Here's how the part is built. I have some questions about the finished solid (model axes, mm). Face numbers are marked on the shaded views. A direction names the side the tool comes from. Coordinates: 2 decimals unless noted, no trailing zeros. Loops run counter-clockwise (first coordinate to the right, second up) from the corner with the lowest first, then second, coordinate; pieces in that order, holes last. Notation, with made-up numbers: M 35,23.25 L 63,23.25 A25 ccw 63,62.25 Z; hole C 7,-13.5 d11. An arc over 180 degrees is marked long. Use CSV: the item, a comma, the result in double quotes. Start each with the question number.
Q1. If we section it at D-D (z = 2.75): Please give me the cut outline in (x, y).
Q2. Which directions (+Z, -Z, +X, -X, +Y, -Y) give clear straight access to the entire face, cutting with the end or side of a thin tool? Please do the marked faces 1 and 2.
Q3. If we section it at C-C (y = 6.25): Please give me the cut outline in (x, z) (3 decimals), and give its area (3 significant figures).
Q4. If we section it at A-A (y = 3.5): Please give me the cut outline in (x, z) (3 decimals), and give its area (3 significant figures).
Q5. If we mould it in two halves opening along Y, with no side actions, what happens to the marked faces 3, 4 and 5? For each: +Y half, -Y half, draft (parallel to the pull), parting line (faces both ways), or undercut.
Q6. For pin 1 Ø3.5 at (y, z) = (5, 16.5) entering from -X; pin 2 Ø5 at (x, y) = (6.5, 4) entering from +Z; pin 3 Ø2.5 at (x, z) = (36.5, 3.5) entering from +Y, each with a flat end and sliding along its axis, tell me the tip position at first contact or that it passes through.
Q7. Please list where these lines run through material, in increasing order: probe 1 along Z at (x, y) = (36.5, 5.5) (3 decimals); probe 2 along Z at (x, y) = (36.5, 6.5) (3 decimals); probe 3 along X at (y, z) = (3.5, 5.75). Write a range as [from, to].
Q8. If we section it at B-B (x = 36.5): Please give me the cut outline in (y, z) (3 decimals), and give its area (3 significant figures).
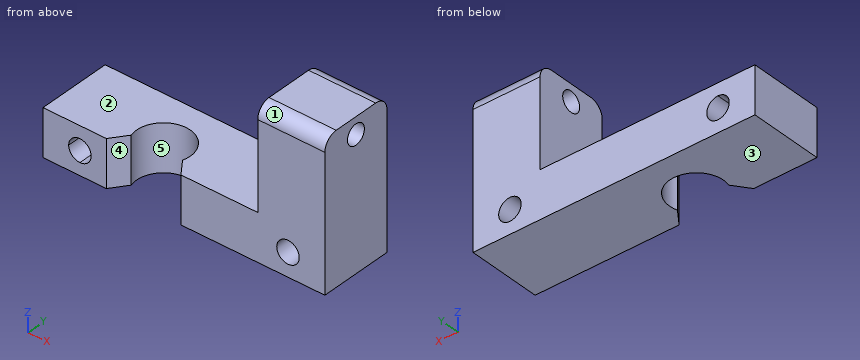
from build123d import *

# Parameters (mm, degrees)
F1_W        = 42
F1_H        = 11
F2_DEPTH    = 7
F3_R        = 4
F4_DEPTH    = 25
F5_T1_DEPTH = 25.9605224852
F7_DEPTH    = 25
F8_W        = 10
F8_H        = 11
F9_DEPTH    = 15
F10_R       = 1.5
F11_DEPTH   = 25
F12_R       = 2


# Not quite as in the source:
# - a fillet or chamfer that OpenCascade refuses, or shapes differently, is made with other operations: its cross-section is extruded or revolved along the edge and cut away or added


with BuildPart() as f2:
    # F1 (on Top) → F2 (new body)
    with BuildSketch(Plane.XY):
        with Locations((21, 5.5)):
            Rectangle(F1_W, F1_H)
    extrude(amount=F2_DEPTH)

    # F3 (on face) → F4 (cut)
    with BuildSketch(Plane.XY.offset(7)):
        with Locations((15, 3.5)):
            Circle(F3_R)
    extrude(amount=-F4_DEPTH, mode=Mode.SUBTRACT)

    # F5: chamfer of 7 on 2 edges, made by hand

    # F5_s2 → F5_t1 (cut)
    with BuildSketch(Plane.XY.offset(-9.4802612426)):
        with BuildLine():
            Line((20.721915214, -0.225000294), (18.6596772309, 2.5591704653))
            Line((18.6596772309, 2.5591704653), (18.5257555, 2.5999745093))
            ThreePointArc((18.5257555, 2.5999745093), (18.0236462707, 1.1005910665), (16.8687144645, 0.1225))
            Line((16.8687144645, 0.1225), (16.9364916731, -0.14))
            ThreePointArc((16.9364916731, -0.14), (18.8292034436, -0.14), (20.721915214, -0.365000294))
            Line((20.721915214, -0.365000294), (20.721915214, -0.225000294))
        make_face()
        with BuildLine():
            Line((11.3403227691, 2.5591704653), (9.278084786, -0.225000294))
            Line((9.278084786, -0.225000294), (9.278084786, -0.365000294))
            ThreePointArc((9.278084786, -0.365000294), (11.1707965564, -0.14), (13.0635083269, -0.14))
            Line((13.0635083269, -0.14), (13.1312855355, 0.1225))
            ThreePointArc((13.1312855355, 0.1225), (11.9763537293, 1.1005910665), (11.4742445, 2.5999745093))
            Line((11.4742445, 2.5999745093), (11.3403227691, 2.5591704653))
        make_face()
    extrude(amount=F5_T1_DEPTH, mode=Mode.SUBTRACT)

    # F6 (on face) → F7 (cut)
    with BuildSketch(Plane(origin=(0, 11, 0), x_dir=(-1, 0, 0), z_dir=(0, 1, 0))):
        with BuildLine():
            Line((-5.5, 3.5), (-3.825, 3.5))
            ThreePointArc((-3.825, 3.5), (-4.3155961415, 4.6844038585), (-5.5, 5.175))
            Line((-5.5, 5.175), (-5.5, 3.5))
        make_face()
        with BuildLine():
            ThreePointArc((-5.5, 1.825), (-4.3155961415, 2.3155961415), (-3.825, 3.5))
            Line((-3.825, 3.5), (-5.5, 3.5))
            Line((-5.5, 3.5), (-5.5, 1.825))
        make_face()
        with BuildLine():
            Line((-5.5, 3.5), (-5.5, 5.175))
            ThreePointArc((-5.5, 5.175), (-7.175, 3.5), (-5.5, 1.825))
            Line((-5.5, 1.825), (-5.5, 3.5))
        make_face()
        with BuildLine():
            ThreePointArc((-38.175, 3.5), (-36.5, 1.825), (-34.825, 3.5))
            ThreePointArc((-34.825, 3.5), (-36.5, 5.175), (-38.175, 3.5))
        make_face()
    extrude(amount=-F7_DEPTH, mode=Mode.SUBTRACT)

    # F8 (on face) → F9 (join)
    with BuildSketch(Plane.XY.offset(7)):
        with Locations((37, 5.5)):
            Rectangle(F8_W, F8_H)
    extrude(amount=F9_DEPTH)

    # F10 (on face) → F11 (cut)
    with BuildSketch(Plane.YZ.offset(42)):
        with Locations((5.5, 19.5)):
            Circle(F10_R)
    extrude(amount=-F11_DEPTH, mode=Mode.SUBTRACT)

    # F12
    f12_edges = [f2.edges().sort_by_distance(p)[0] for p in [
        (37, 0, 22),
        (37, 11, 22),
    ]]
    fillet(f12_edges, radius=F12_R)


solid = f2.part
Results below:
1,outline,"M 0,0 L 4,0 L 4,11 L 0,11 Z; M 7,0 L 9.44,0 L 11.17,2.33 A4 cw long 18.83,2.33 L 20.56,0 L 35,0 L 35,11 L 7,11 Z; M 38,0 L 42,0 L 42,11 L 38,11 Z"
2,face 1,"+Z, +X, -X, -Y"
2,face 2,"+Z, -X, +Y, -Y"
3,outline,"M 0,0 L 12.095,0 L 12.095,7 L 0,7 Z; M 17.905,0 L 42,0 L 42,18.201 L 32,18.201 L 32,7 L 17.905,7 Z; M 32,20.799 L 42,20.799 L 42,22 L 32,22 Z; hole C 5.5,3.5 d3.35; hole C 36.5,3.5 d3.35"
3,area,"360 mm^2"
4,outline,"M 0,0 L 11,0 L 11,7 L 0,7 Z; M 19,0 L 42,0 L 42,22 L 32,22 L 32,7 L 19,7 Z; hole C 5.5,3.5 d3.35; hole C 36.5,3.5 d3.35"
4,area,"370 mm^2"
5,face 3,"draft"
5,face 4,"-Y half"
5,face 5,"undercut"
6,pin 1,"x = 32"
6,pin 2,"z = 7"
6,pin 3,"through"
7,probe 1,"[0, 1.825], [5.175, 18], [21, 22]"
7,probe 2,"[0, 1.825], [5.175, 18.382], [20.618, 22]"
7,probe 3,"[0, 11], [19, 42]"
8,outline,"M 0,0 L 11,0 L 11,1.825 L 0,1.825 Z; M 0,5.175 L 11,5.175 L 11,20 A2 ccw 9,22 L 2,22 A2 ccw 0,20 Z; hole C 5.5,19.5 d3"
8,area,"196 mm^2"
